Drawing for the job (mm, zero at the part's lowest x, y, z). A direction names the side the tool comes from. Give positions to 0.01 mm unless a question says otherwise; leave off trailing zeros. Order: outer loops, then holes, each group sorted by start corner. A loop starts at its lowest first (then second) coordinate and runs counter-clockwise, first axis right, second up. Notation, with made-up numbers: (-18.5, -13.75) - (-0.5, -13.75) arc R20 cw to (-0.5, -0.75) - close; hole circle Ø8 at (1.25, -21.5). An arc over 180 degrees is marked (long way). One line per item, written item: value.
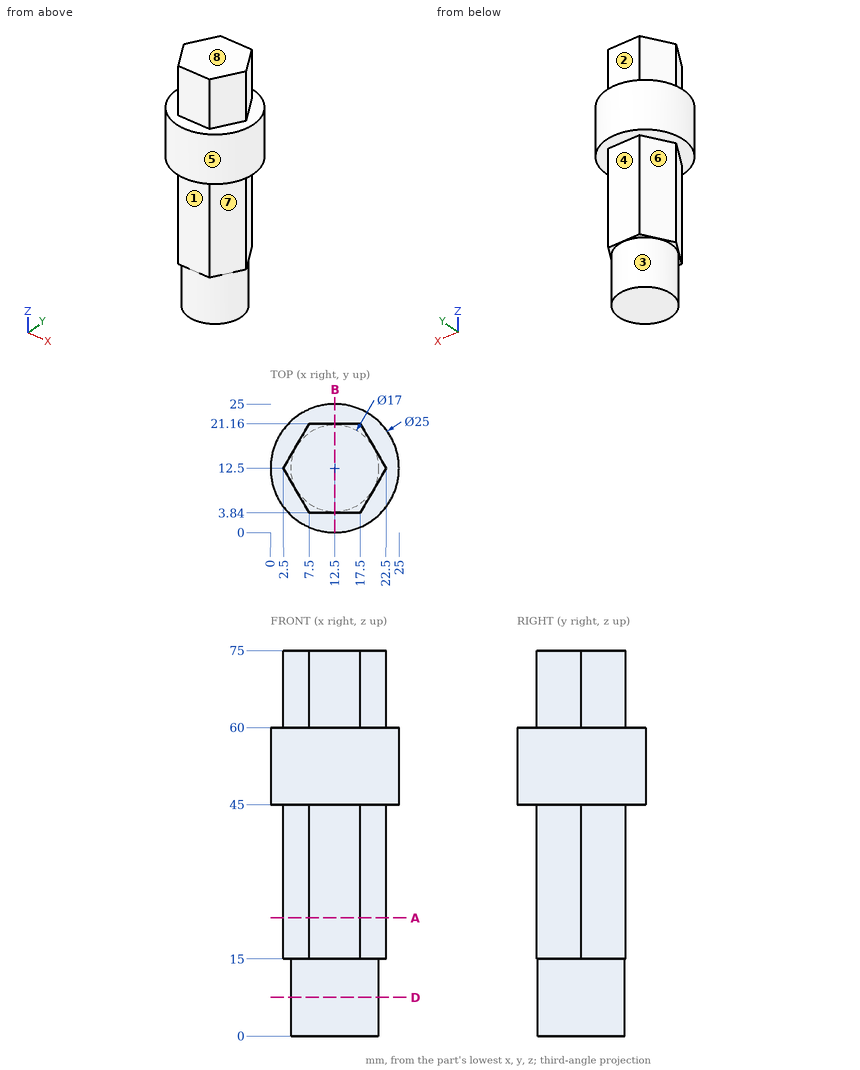
1) Mould opens along X. For the marked faces 5, 6, 7 and 8 say: released by +X, released by -X, zero draft, split by the parting line, or undercut.
Outcome:
face 5: split by the parting line
face 6: released by -X
face 7: released by +X
face 8: zero draft
2) Drill centre lines: line 1 along Z through (x, y) = (7.25, 4.5); line 2 along Y through (x, z) = (8.25, 62); line 3 along Z through (x, y) = (10.5, 2). Where is each one in solid material? Low to high. Write a range as from..to.
Outcome:
line 1: z = 15..75
line 2: y = 3.84..21.16
line 3: z = 45..60
3) Cut at A-A, the plane z = 23. Give the cut face in (x, y).
Outcome:
outline: (2.5, 12.5) - (7.5, 3.84) - (17.5, 3.84) - (22.5, 12.5) - (17.5, 21.16) - (7.5, 21.16) - close
4) Cut at B-B, the plane x = 12.5. Give the cut face in (y, z), then the cut area to 3 significant figures.
Outcome:
outline: (0, 45) - (3.84, 45) - (3.84, 15) - (4, 15) - (4, 0) - (21, 0) - (21, 15) - (21.16, 15) - (21.16, 45) - (25, 45) - (25, 60) - (21.16, 60) - (21.16, 75) - (3.84, 75) - (3.84, 60) - (0, 60) - close
area: 1,410 mm^2
5) Cut at D-D, the plane z = 7.5. Give the cut face in (x, y).
Outcome:
outline: circle Ø17 at (12.5, 12.5)
6) Pin check, flat tips, straight feed: pin 1 (3 mm diameter, centred on y = 21.5, z = 48.5, fed in from +X); pin 2 (3 mm diameter, centred on x = 21.5, z = 9, fed in from +Y); pin 3 (8 mm diameter, centred on x = 14, z = 28, fed in from -Y). Stop position of each tip, or through.
Outcome:
pin 1: stops at x = 22.5
pin 2: stops at y = 16.5
pin 3: stops at y = 3.84
7) Which spindle directions (+Z, -Z, +X, -X, +Y, -Y) get a long thin tool onto all of the face, cutting with end or side? Do the marked faces 1, 2, 3 and 4. Say none if no direction does.
Outcome:
face 1: -Z, +X, -X, -Y
face 2: +Z, +X, -X, +Y
face 3: -Z
face 4: -Z, +X, -X, +Y
